Can you work these out from the drawing? Everything is in mm from the part's minimum corner. Give positions to 0.01 mm unless a question says otherwise; leave off trailing zeros. Write each loop counter-clockwise with the first axis right and the second up, starting at its lowest first coordinate (ties: lowest second). Pieces come first, ordered by that corner, then holes. Notation, with made-up numbers: (80, 63.5) - (96, 63.5) arc R26 cw to (96, 97.5) - close; hole circle Ø6 at (-34.5, 33.5). An arc over 180 degrees is marked (long way). Write each question's results on one line, items separated by ' | '. Start each with the question number.
Item 1: Suppose I cut it at C-C on z = 0.9. List the corners of the cut face in (x, y) for me, then the cut area to 3 significant figures.
Item 2: Suppose I cut it at A-A on x = 2.5. List the corners of the cut face in (y, z) for me, then the cut area to 3 significant figures.
Item 3: Please list where these lines run through material, in increasing order: line 1 along X through (y, z) = (28, 1.3); line 2 along Y through (x, z) = (2.5, 0.4); line 3 along X through (y, z) = (27, 2.45).
Item 4: Suppose I cut it at B-B on y = 28.09. List the corners of the cut face in (x, z) for me.
Item 5: Will these pins go through, and if not, where does the flat tip stop? P1, Ø1.6, axis at x = 36.5, y = 28.09, coming from the -Z side; P2, Ø1.2, axis at x = 36, y = 2, coming from the +Z side.
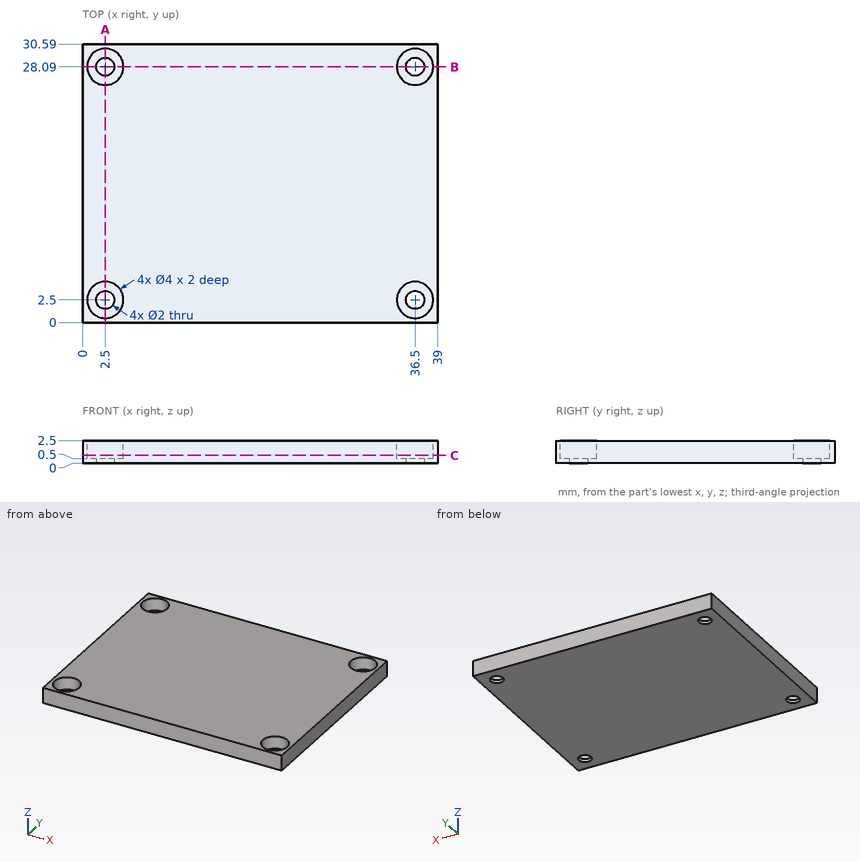
Checked values:
1) outline: (0, 0) - (39, 0) - (39, 30.59) - (0, 30.59) - close; hole circle Ø4 at (2.5, 2.5); hole circle Ø4 at (2.5, 28.09); hole circle Ø4 at (36.5, 2.5); hole circle Ø4 at (36.5, 28.09) | area: 1,140 mm^2
2) outline: (0, 0) - (1.5, 0) - (1.5, 0.5) - (0.5, 0.5) - (0.5, 2.5) - (0, 2.5) - close; (3.5, 0) - (27.09, 0) - (27.09, 0.5) - (26.09, 0.5) - (26.09, 2.5) - (4.5, 2.5) - (4.5, 0.5) - (3.5, 0.5) - close; (29.09, 0) - (30.59, 0) - (30.59, 2.5) - (30.09, 2.5) - (30.09, 0.5) - (29.09, 0.5) - close | area: 58.5 mm^2
3) line 1: x = 0 to 0.5, 4.5 to 34.5, 38.5 to 39 | line 2: y = 0 to 1.5, 3.5 to 27.09, 29.09 to 30.59 | line 3: x = 0 to 0.82, 4.18 to 34.82, 38.18 to 39
4) outline: (0, 0) - (1.5, 0) - (1.5, 0.5) - (0.5, 0.5) - (0.5, 2.5) - (0, 2.5) - close; (3.5, 0) - (35.5, 0) - (35.5, 0.5) - (34.5, 0.5) - (34.5, 2.5) - (4.5, 2.5) - (4.5, 0.5) - (3.5, 0.5) - close; (37.5, 0) - (39, 0) - (39, 2.5) - (38.5, 2.5) - (38.5, 0.5) - (37.5, 0.5) - close
5) P1: passes through | P2: stops at z = 0.5
